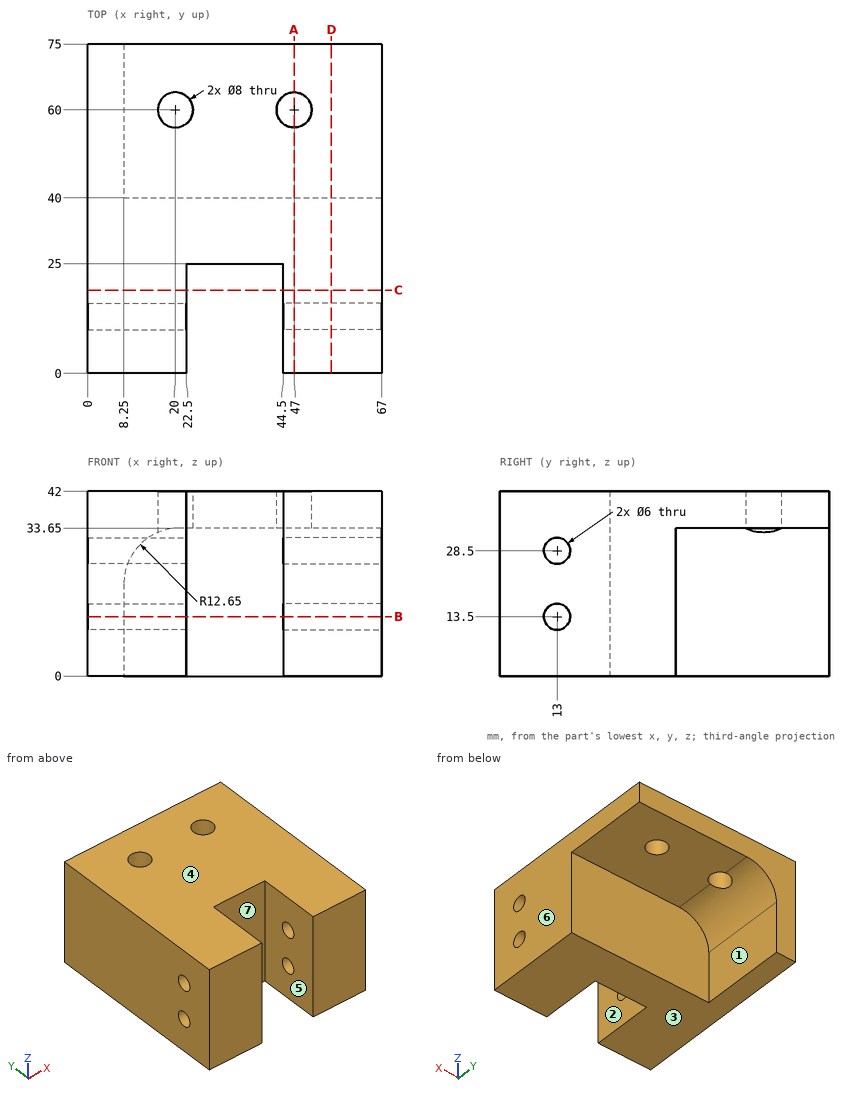
Check sheet for the drawn part. Datum: minimum x, y, z corner. Units: mm. A direction names the side the tool comes from. Coordinates: 2 decimals unless noted, no trailing zeros. Loops run counter-clockwise (first coordinate to the right, second up) from the corner with the lowest first, then second, coordinate; pieces in that order, holes last. Notation, with made-up numbers: (-33, 60) -> (-25, 60) arc R30 cw to (-25, 98) -> close; hole circle Ø6 at (-29, -21.75). An arc over 180 degrees is marked (long way). Answer in a Markdown table with one row per item.
1) Section check B-B (z = 13.5). Record the cut outline in (x, y), and give its area (3 significant figures).
The answers:
| item | result |
|---|---|
| outline | (0, 0) -> (22.5, 0) -> (22.5, 10) -> (0, 10) -> close; (0, 16) -> (22.5, 16) -> (22.5, 25) -> (44.5, 25) -> (44.5, 16) -> (67, 16) -> (67, 40) -> (8.25, 40) -> (8.25, 75) -> (0, 75) -> close; (44.5, 0) -> (67, 0) -> (67, 10) -> (44.5, 10) -> close |
| area | 2,150 mm2 |
2) Section check A-A (x = 47). Record the cut outline in (y, z).
The answers:
| item | result |
|---|---|
| outline | (0, 0) -> (40, 0) -> (40, 33.65) -> (56, 33.65) -> (56, 42) -> (0, 42) -> close; (64, 33.65) -> (75, 33.65) -> (75, 42) -> (64, 42) -> close; hole circle Ø6 at (13, 13.5); hole circle Ø6 at (13, 28.5) |
3) Section check C-C (y = 19). Record the cut outline in (x, z).
The answers:
| item | result |
|---|---|
| outline | (0, 0) -> (22.5, 0) -> (22.5, 42) -> (0, 42) -> close; (44.5, 0) -> (67, 0) -> (67, 42) -> (44.5, 42) -> close |
4) Section check D-D (x = 55.5). Record the cut outline in (y, z).
The answers:
| item | result |
|---|---|
| outline | (0, 0) -> (40, 0) -> (40, 33.65) -> (75, 33.65) -> (75, 42) -> (0, 42) -> close; hole circle Ø6 at (13, 13.5); hole circle Ø6 at (13, 28.5) |
5) Depth check by flat-ended pin: P1, Ø17.5, axis at x = 47, y = 54, coming from the -Z side; P2, Ø17, axis at x = 39.5, z = 10, coming from the +Y side; P3, Ø23, axis at y = 58, z = 7.5, coming from the +X side. Enter the tip coordinate at first touch or a pass-through.
The answers:
| item | result |
|---|---|
| P1 | stops at z = 33.65 |
| P2 | stops at y = 40 |
| P3 | stops at x = 8.25 |
6) Scan lines: line 1 along X through (y, z) = (4.5, 4); line 2 along Y through (x, z) = (8.75, 28.5); line 3 along Y through (x, z) = (47, 37). Record each from-to range of solid material in increasing order. Write a range as from..to.
The answers:
| item | result |
|---|---|
| line 1 | x = 0..22.5, 44.5..67 |
| line 2 | y = 0..10, 16..75 |
| line 3 | y = 0..56, 64..75 |
7) Draft check along X on the marked faces 4, 5, 6 and 7. Enter one of: released by +X, released by -X, zero draft, split by the parting line, or undercut.
The answers:
| item | result |
|---|---|
| face 4 | zero draft |
| face 5 | undercut |
| face 6 | released by +X |
| face 7 | undercut |
8) Access from +Z, -Z, +X, -X, +Y, -Y to the whole of each face (thin tool, end or side, straight path). Record for the marked faces 1, 2 and 3.
The answers:
| item | result |
|---|---|
| face 1 | -Z, +X, +Y |
| face 2 | +Z, -Z, -Y |
| face 3 | -Z, +X, -X, +Y, -Y |
